Check sheet for the modelled part. Datum: model origin and axes. Units: mm. A direction names the side the tool comes from. Coordinates: 2 decimals unless noted, no trailing zeros. Write each loop counter-clockwise with the first axis right and the second up, starting at its lowest first coordinate (ties: lowest second). Pieces come first, ordered by that corner, then holes. Notation, with made-up numbers: (-38, -8.5) - (-28, -8.5) arc R26 cw to (-28, 29.5) - close; hole circle Ø8 at (17.5, 28.5). An arc over 180 degrees is marked (long way). Write each question's results on one line, items separated by ' | '.
from build123d import *

# Parameters (mm, degrees)
SZKIC1_W                    = 10
SZKIC1_H                    = 178
DODANIE_WYCI_GNI_CIE1_DEPTH = 490
WYTNIJ_WYCI_GNI_CIE1_DEPTH  = 522.424970633
WYTNIJ_WYCI_GNI_CIE2_DEPTH  = 522.424970633
ZAOKR_GLENIE1_R             = 100
ZAOKR_GLENIE2_R             = 100
WYTNIJ_WYCI_GNI_CIE3_DEPTH  = 522.424970633
ZAOKR_GLENIE3_R             = 10
SZKIC6_W                    = 60
SZKIC6_H                    = 10
DODANIE_WYCI_GNI_CIE2_DEPTH = 490
ZAOKR_GLENIE4_R             = 5
ZAOKR_GLENIE5_R             = 4
ZAOKR_GLENIE6_R             = 5
WYTNIJ_WYCI_GNI_CIE4_DEPTH  = 10
WYTNIJ_WYCI_GNI_CIE5_DEPTH  = 10
WYTNIJ_WYCI_GNI_CIE6_DEPTH  = 10


with BuildPart() as part:
    # Szkic1 → Dodanie-wyciągnięcie1 (new body)
    with BuildSketch(Plane.XY):
        with Locations((-5, 89)):
            Rectangle(SZKIC1_W, SZKIC1_H)
    extrude(amount=DODANIE_WYCI_GNI_CIE1_DEPTH)

    # Szkic2 → Wytnij-wyciągnięcie1 (cut, through all)
    with BuildSketch(Plane(origin=(0, 0, 0), x_dir=(0, 0, -1), z_dir=(1, 0, 0))):
        with BuildLine():
            Line((-107.5, 168), (-92.5, 168))
            ThreePointArc((-92.5, 168), (-82.5, 158), (-92.5, 148))
            Line((-92.5, 148), (-107.5, 148))
            ThreePointArc((-107.5, 148), (-117.5, 158), (-107.5, 168))
        make_face()
        with BuildLine():
            Line((-107.5, 138), (-92.5, 138))
            ThreePointArc((-92.5, 138), (-82.5, 128), (-92.5, 118))
            Line((-92.5, 118), (-107.5, 118))
            ThreePointArc((-107.5, 118), (-117.5, 128), (-107.5, 138))
        make_face()
        with BuildLine():
            Line((-107.5, 108), (-92.5, 108))
            ThreePointArc((-92.5, 108), (-82.5, 98), (-92.5, 88))
            Line((-92.5, 88), (-107.5, 88))
            ThreePointArc((-107.5, 88), (-117.5, 98), (-107.5, 108))
        make_face()
        with BuildLine():
            Line((-107.5, 78), (-92.5, 78))
            ThreePointArc((-92.5, 78), (-82.5, 68), (-92.5, 58))
            Line((-92.5, 58), (-107.5, 58))
            ThreePointArc((-107.5, 58), (-117.5, 68), (-107.5, 78))
        make_face()
        with BuildLine():
            Line((-107.5, 48), (-92.5, 48))
            ThreePointArc((-92.5, 48), (-82.5, 38), (-92.5, 28))
            Line((-92.5, 28), (-107.5, 28))
            ThreePointArc((-107.5, 28), (-117.5, 38), (-107.5, 48))
        make_face()
    extrude(amount=-WYTNIJ_WYCI_GNI_CIE1_DEPTH, mode=Mode.SUBTRACT)

    # Szkic3 → Wytnij-wyciągnięcie2 (cut, through all)
    with BuildSketch(Plane(origin=(0, 0, 0), x_dir=(0, 0, -1), z_dir=(1, 0, 0))):
        with BuildLine():
            Line((-397.5, 168), (-382.5, 168))
            ThreePointArc((-382.5, 168), (-372.5, 158), (-382.5, 148))
            Line((-382.5, 148), (-397.5, 148))
            ThreePointArc((-397.5, 148), (-407.5, 158), (-397.5, 168))
        make_face()
        with BuildLine():
            Line((-397.5, 138), (-382.5, 138))
            ThreePointArc((-382.5, 138), (-372.5, 128), (-382.5, 118))
            Line((-382.5, 118), (-397.5, 118))
            ThreePointArc((-397.5, 118), (-407.5, 128), (-397.5, 138))
        make_face()
        with BuildLine():
            Line((-397.5, 108), (-382.5, 108))
            ThreePointArc((-382.5, 108), (-372.5, 98), (-382.5, 88))
            Line((-382.5, 88), (-397.5, 88))
            ThreePointArc((-397.5, 88), (-407.5, 98), (-397.5, 108))
        make_face()
        with BuildLine():
            Line((-397.5, 78), (-382.5, 78))
            ThreePointArc((-382.5, 78), (-372.5, 68), (-382.5, 58))
            Line((-382.5, 58), (-397.5, 58))
            ThreePointArc((-397.5, 58), (-407.5, 68), (-397.5, 78))
        make_face()
        with BuildLine():
            Line((-397.5, 48), (-382.5, 48))
            ThreePointArc((-382.5, 48), (-372.5, 38), (-382.5, 28))
            Line((-382.5, 28), (-397.5, 28))
            ThreePointArc((-397.5, 28), (-407.5, 38), (-397.5, 48))
        make_face()
    extrude(amount=-WYTNIJ_WYCI_GNI_CIE2_DEPTH, mode=Mode.SUBTRACT)

    # Zaokrąglenie1
    zaokr_glenie1_edges = [part.edges().sort_by_distance(p)[0] for p in [
        (-5, 178, 0),
    ]]
    fillet(zaokr_glenie1_edges, radius=ZAOKR_GLENIE1_R)

    # Zaokrąglenie2
    zaokr_glenie2_edges = [part.edges().sort_by_distance(p)[0] for p in [
        (-5, 178, 490),
    ]]
    fillet(zaokr_glenie2_edges, radius=ZAOKR_GLENIE2_R)

    # Szkic5 → Wytnij-wyciągnięcie3 (cut, through all)
    with BuildSketch(Plane.ZY.offset(10)):
        with BuildLine():
            Line((136.235236097, 178), (353.764763903, 178))
            ThreePointArc((353.764763903, 178), (245, 69.235236097), (136.235236097, 178))
        make_face()
    extrude(amount=-WYTNIJ_WYCI_GNI_CIE3_DEPTH, mode=Mode.SUBTRACT)

    # Zaokrąglenie3
    zaokr_glenie3_edges = [part.edges().sort_by_distance(p)[0] for p in [
        (-5, 178, 353.764763903),
        (-5, 178, 136.235236097),
    ]]
    fillet(zaokr_glenie3_edges, radius=ZAOKR_GLENIE3_R)

    # Szkic6 → Dodanie-wyciągnięcie2 (add, through all)
    with BuildSketch(Plane(origin=(0, 0, 0), x_dir=(-1, 0, 0), z_dir=(0, 0, -1))):
        with Locations((-20, 5)):
            Rectangle(SZKIC6_W, SZKIC6_H)
    extrude(amount=-DODANIE_WYCI_GNI_CIE2_DEPTH)

    # Zaokrąglenie4
    zaokr_glenie4_edges = [part.edges().sort_by_distance(p)[0] for p in [
        (-10, 0, 245),
    ]]
    fillet(zaokr_glenie4_edges, radius=ZAOKR_GLENIE4_R)

    # Zaokrąglenie5
    zaokr_glenie5_edges = [part.edges().sort_by_distance(p)[0] for p in [
        (0, 10, 245),
    ]]
    fillet(zaokr_glenie5_edges, radius=ZAOKR_GLENIE5_R)

    # Zaokrąglenie6
    zaokr_glenie6_edges = [part.edges().sort_by_distance(p)[0] for p in [
        (50, 5, 0),
        (50, 5, 490),
    ]]
    fillet(zaokr_glenie6_edges, radius=ZAOKR_GLENIE6_R)

    # Szkic7 → Wytnij-wyciągnięcie4 (cut)
    with BuildSketch(Plane(origin=(0, 10, 0), x_dir=(1, 0, 0), z_dir=(0, 1, 0))):
        with BuildLine():
            Line((32.5, -468.6), (17.5, -468.6))
            ThreePointArc((17.5, -468.6), (8.9, -460), (17.5, -451.4))
            Line((17.5, -451.4), (32.5, -451.4))
            ThreePointArc((32.5, -451.4), (41.1, -460), (32.5, -468.6))
        make_face()
    wytnij_wyci_gni_cie4 = extrude(amount=-WYTNIJ_WYCI_GNI_CIE4_DEPTH, mode=Mode.SUBTRACT)

    # Lustro2: Wytnij-wyciągnięcie4 across plane
    add(wytnij_wyci_gni_cie4.mirror(Plane(origin=(0, 0, 245), x_dir=(1, 0, 0), z_dir=(0, 0, -1))), mode=Mode.SUBTRACT)

    # Szkic8 → Wytnij-wyciągnięcie5 (cut)
    with BuildSketch(Plane(origin=(0, 10, 0), x_dir=(1, 0, 0), z_dir=(0, 1, 0))):
        with BuildLine():
            Line((17.5, -421.4), (32.5, -421.4))
            ThreePointArc((32.5, -421.4), (41.1, -430), (32.5, -438.6))
            Line((32.5, -438.6), (17.5, -438.6))
            ThreePointArc((17.5, -438.6), (8.9, -430), (17.5, -421.4))
        make_face()
    wytnij_wyci_gni_cie5 = extrude(amount=-WYTNIJ_WYCI_GNI_CIE5_DEPTH, mode=Mode.SUBTRACT)

    # Lustro3: Wytnij-wyciągnięcie5 across plane
    add(wytnij_wyci_gni_cie5.mirror(Plane(origin=(0, 0, 245), x_dir=(1, 0, 0), z_dir=(0, 0, -1))), mode=Mode.SUBTRACT)

    # Szkic9 → Wytnij-wyciągnięcie6 (cut)
    with BuildSketch(Plane(origin=(0, 10, 0), x_dir=(1, 0, 0), z_dir=(0, 1, 0))):
        with BuildLine():
            Line((17.5, -391.4), (32.5, -391.4))
            ThreePointArc((32.5, -391.4), (41.1, -400), (32.5, -408.6))
            Line((32.5, -408.6), (17.5, -408.6))
            ThreePointArc((17.5, -408.6), (8.9, -400), (17.5, -391.4))
        make_face()
    wytnij_wyci_gni_cie6 = extrude(amount=-WYTNIJ_WYCI_GNI_CIE6_DEPTH, mode=Mode.SUBTRACT)

    # Lustro4: Wytnij-wyciągnięcie6 across plane
    add(wytnij_wyci_gni_cie6.mirror(Plane(origin=(0, 0, 245), x_dir=(1, 0, 0), z_dir=(0, 0, -1))), mode=Mode.SUBTRACT)


solid = part.part
1. Go/stop test with flat-tipped pins: pin 1 (5 mm diameter, centred on x = -7, z = 101, fed in from -Y); pin 2 (3 mm diameter, centred on x = -7.5, z = 96.5, fed in from +Y); pin 3 (1 mm diameter, centred on y = 116, z = 78, fed in from +X); pin 4 (3 mm diameter, centred on x = 5, z = 147.5, fed in from +Y). Record where each tip stops, or that it passes through.
Values follow:
pin 1: stops at y = 0 | pin 2: stops at y = 177.98 | pin 3: stops at x = 0 | pin 4: stops at y = 10.03
2. Access from +Z, -Z, +X, -X, +Y, -Y to the whole of each face (thin tool, end or side, straight path). Record for faces 1 (the flat face through (-5, 168, 100)), 2 (the cylindrical face through (8.902, 5.07, 430.189)), 3 (the flat face through (-1, 28, 490)).
Values follow:
face 1: +X, -X | face 2: +Y, -Y | face 3: +Z, +X, -X, +Y, -Y
3. Draft check along Y on faces 4 (the cylindrical face through (-4.9, 38.2, 82.5)), 5 (the cylindrical face through (-5.07, 69.26, 247.26)), 6 (the flat face through (0, 58, 242)). Enter one of: pulls with the +Y half, pulls with the -Y half, needs draft (parallel to the pull), parting line crosses it, or undercut.
Values follow:
face 4: undercut | face 5: pulls with the +Y half | face 6: needs draft
4. Sectioned sample at C-C (y = 158). Record the cut outline in (x, z).
Values follow:
outline: (-10, 40) - (0, 40) - (0, 82.5) - (-10, 82.5) - close; (-10, 117.5) - (0, 117.5) - (0, 138.09) - (-10, 138.09) - close; (-10, 351.91) - (0, 351.91) - (0, 372.5) - (-10, 372.5) - close; (-10, 407.5) - (0, 407.5) - (0, 450) - (-10, 450) - close
5. Material ranges on L1, parallel to Z at x = -0.5, y = 149; L2, parallel to Z at x = -3, y = 36.5; L3, parallel to Y at x = 34.5, z = 359, recorded low to high. Write a range as [from, to].
Values follow:
L1: z = [29.58, 88.14], [111.86, 140.17], [349.83, 378.14], [401.86, 460.42] | L2: z = [0, 82.61], [117.39, 372.61], [407.39, 490] | L3: y = [0, 10]
6. Sectioned sample at A-A (y = 38). Record the cut outline in (x, z), then the cut area to 3 significant figures.
Values follow:
outline: (-10, 0) - (0, 0) - (0, 82.5) - (-10, 82.5) - close; (-10, 117.5) - (0, 117.5) - (0, 372.5) - (-10, 372.5) - close; (-10, 407.5) - (0, 407.5) - (0, 490) - (-10, 490) - close | area: 4,200 mm^2
7. Sectioned sample at D-D (z = 255). Record the cut outline in (x, y).
Values follow:
outline: (-10, 5) arc R5 ccw to (-5, 0) - (50, 0) - (50, 10) - (4, 10) arc R4 cw to (0, 14) - (0, 69.7) - (-10, 69.7) - close
8. Sectioned sample at B-B (z = 30). Record the cut outline in (x, y).
Values follow:
outline: (-10, 5) arc R5 ccw to (-5, 0) - (8.9, 0) - (8.9, 10) - (4, 10) arc R4 cw to (0, 14) - (0, 149.41) - (-10, 149.41) - close; (41.1, 0) - (50, 0) - (50, 10) - (41.1, 10) - close
